Part model, mm, in its own coordinate system. A direction names the side the tool comes from. Coordinates: 2 decimals unless noted, no trailing zeros. Loops run counter-clockwise (first coordinate to the right, second up) from the corner with the lowest first, then second, coordinate; pieces in that order, holes last. Notation, with made-up numbers: M 47.25,46 L 69.25,46 A15 ccw 69.25,57 Z; hole C 86,16 d11. An arc over 180 degrees is marked long. Use a Markdown table: item, result. Add a question column.
1) Wall check: probe 1 along Y at (x, z) = (-881, 10.5). Give the ranges that are in metal, low to high. Write a range as from..to.
2) Band-saw the part on A-A (z = 17.5). List the corners of the cut face in (x, y).
3) Band-saw the part on B-B (x = -754). List the corners of the cut face in (y, z), plus the area to 3 significant figures.
4) Tool access for faces 1 (the flat face through (-732, -208, 10)), 2 (the flat face through (-802, -295, 0)), 3 (the flat face through (-877, -197, 10)): list every direction of +Z, -Z, +X, -X, +Y, -Y with a clear straight run to the whole face (end or side of a thin tool).
from build123d import *

# Parameters (mm, degrees)
F3_DEPTH  = 240
F5_DEPTH  = 20
F6_W      = 112
F6_H      = 241.1060750484
F7_DEPTH  = 25
F8_W      = 70.001994
F8_H      = 85
F9_DEPTH  = 25
F10_W     = 50
F10_H     = 198.001994
F11_DEPTH = 50
F12_DEPTH = 240.001
F13_DEPTH = 70.001


with BuildPart() as f3:
    # F2 (on face) → F3 (new body)
    with BuildSketch(Plane.XY):
        Polygon((-627, -343.001994), (-627, -273), (-627, -187), (-765, -187), (-877, -187), (-925, -187), (-925, -427.001994), (-627, -427.001994), align=None)
        Polygon((-765, -208), (-648, -208), (-648, -273), (-648, -343.001994), (-648, -406.001994), (-904, -406.001994), (-904, -208), (-877, -208), align=None, mode=Mode.SUBTRACT)
    extrude(amount=F3_DEPTH)

    # F4 (on face) → F5 (join)
    with BuildSketch(Plane.XY):
        Polygon((-648, -273), (-648, -208), (-765, -208), (-877, -208), (-904, -208), (-904, -406.001994), (-648, -406.001994), (-648, -343.001994), align=None)
    extrude(amount=F5_DEPTH)

    # F6 (on face) → F7 (cut)
    with BuildSketch(Plane(origin=(0, -187, 0), x_dir=(-1, 0, 0), z_dir=(0, 1, 0))):
        with Locations((821, 140.5530375242)):
            Rectangle(F6_W, F6_H)
    extrude(amount=-F7_DEPTH, mode=Mode.SUBTRACT)

    # F8 (on face) → F9 (cut)
    with BuildSketch(Plane.YZ.offset(-627)):
        with Locations((-308.000997, 177.5)):
            Rectangle(F8_W, F8_H)
    extrude(amount=-F9_DEPTH, mode=Mode.SUBTRACT)

    # F10 (on face) → F11 (join)
    with BuildSketch(Plane.XY.offset(20)):
        with Locations((-673, -307.000997)):
            Rectangle(F10_W, F10_H)
    extrude(amount=F11_DEPTH)

    # F12 (cut, through all): a face of the model
    f12_faces = [f3.faces().sort_by_distance(p)[0] for p in [
        (-630.8262900716, -307.000997, 240),
    ]]
    extrude(f12_faces, amount=-F12_DEPTH, mode=Mode.SUBTRACT)

    # F13 (cut, through all): a face of the model
    f13_faces = [f3.faces().sort_by_distance(p)[0] for p in [
        (-673, -307.000997, 70),
    ]]
    extrude(f13_faces, amount=-F13_DEPTH, mode=Mode.SUBTRACT)


solid = f3.part
Entries:
| question | item | result |
|---|---|---|
| 1 | probe 1 | -406..-208 |
| 2 | outline | M -904,-406 L -698,-406 L -698,-208 L -765,-208 L -765,-187 L -877,-187 L -877,-208 L -904,-208 Z |
| 3 | outline | M -406,0 L -208,0 L -208,20 L -406,20 Z |
| 3 | area | 3,960 mm2 |
| 4 | face 1 | +Z, -Z, +X, +Y |
| 4 | face 2 | -Z, +X, -X, +Y, -Y |
| 4 | face 3 | +Z, -Z, -X, +Y |
